from build123d import *

# Parameters (mm, degrees)
SKETCH_1_R      = 2
EXTRUDE_1_DEPTH = 5
FILLET_2_R      = 2


with BuildPart() as part:
    # 草图1 → 凸台-拉伸1 (new body)
    with BuildSketch(Plane.XY):
        with BuildLine():
            Line((-39, -23.5), (39, -23.5))
            Line((39, -23.5), (39, 46.5))
            Line((39, 46.5), (30.3, 46.5))
            Line((30.3, 46.5), (30.3, 29))
            ThreePointArc((30.3, 29), (0, -1.3), (-30.3, 29))
            Line((-30.3, 29), (-30.3, 46.5))
            Line((-30.3, 46.5), (-39, 46.5))
            Line((-39, 46.5), (-39, -23.5))
        make_face()
        with Locations((-34.65, 39)):
            Circle(SKETCH_1_R, mode=Mode.SUBTRACT)
        with Locations((-34.65, 19)):
            Circle(SKETCH_1_R, mode=Mode.SUBTRACT)
        with Locations((34.65, 19)):
            Circle(SKETCH_1_R, mode=Mode.SUBTRACT)
        with Locations((34.65, 39)):
            Circle(SKETCH_1_R, mode=Mode.SUBTRACT)
        with BuildLine():
            Line((-32, -10.5), (-32, -16.5))
            ThreePointArc((-32, -16.5), (-29, -19.5), (-26, -16.5))
            Line((-26, -16.5), (-26, -10.5))
            ThreePointArc((-26, -10.5), (-29, -7.5), (-32, -10.5))
        make_face(mode=Mode.SUBTRACT)
        with BuildLine():
            Line((26, -10.5), (26, -16.5))
            ThreePointArc((26, -16.5), (29, -19.5), (32, -16.5))
            Line((32, -16.5), (32, -10.5))
            ThreePointArc((32, -10.5), (29, -7.5), (26, -10.5))
        make_face(mode=Mode.SUBTRACT)
    extrude(amount=EXTRUDE_1_DEPTH)

    # 圆角2
    fillet_2_edges = [part.edges().sort_by_distance(p)[0] for p in [
        (30.3, 46.5, 2.5),
        (39, 46.5, 2.5),
        (39, -23.5, 2.5),
        (-39, -23.5, 2.5),
        (-39, 46.5, 2.5),
        (-30.3, 46.5, 2.5),
    ]]
    fillet(fillet_2_edges, radius=FILLET_2_R)


solid = part.part
Check sheet for the modelled part. Datum: model origin and axes. Units: mm. A direction names the side the tool comes from. Coordinates: 2 decimals unless noted, no trailing zeros. Write each loop counter-clockwise with the first axis right and the second up, starting at its lowest first coordinate (ties: lowest second). Pieces come first, ordered by that corner, then holes.
Item 1: Cross-section at A-A on y = -12.5. Record the boundary of the cut face in (x, z), then the cut area to 3 significant figures.
Numbers:
outline: (-39, 0) - (-32, 0) - (-32, 5) - (-39, 5) - close; (-26, 0) - (26, 0) - (26, 5) - (-26, 5) - close; (32, 0) - (39, 0) - (39, 5) - (32, 5) - close
area: 330 mm2
Item 2: Access from +Z, -Z, +X, -X, +Y, -Y to the whole of each face (thin tool, end or side, straight path). Record for faces 5 (the face through (38.43, 45.9, 2.54)), 6 (the face through (28.9, -19.5, 2.5)), 7 (the face through (-30.3, 37, 2)).
Numbers:
face 5: +Z, -Z, +X, +Y
face 6: +Z, -Z
face 7: +Z, -Z, +Y
Item 3: Cross-section at B-B on z = 0.8. Record the boundary of the cut face in (x, y).
Numbers:
outline: (-39, -21.5) arc R2 ccw to (-37, -23.5) - (37, -23.5) arc R2 ccw to (39, -21.5) - (39, 44.5) arc R2 ccw to (37, 46.5) - (32.3, 46.5) arc R2 ccw to (30.3, 44.5) - (30.3, 29) arc R30.3 cw to (-30.3, 29) - (-30.3, 44.5) arc R2 ccw to (-32.3, 46.5) - (-37, 46.5) arc R2 ccw to (-39, 44.5) - close; hole circle Ø4 at (-34.65, 19); hole circle Ø4 at (-34.65, 39); hole (-32, -16.5) arc R3 ccw to (-26, -16.5) - (-26, -10.5) arc R3 ccw to (-32, -10.5) - close; hole (26, -16.5) arc R3 ccw to (32, -16.5) - (32, -10.5) arc R3 ccw to (26, -10.5) - close; hole circle Ø4 at (34.65, 19); hole circle Ø4 at (34.65, 39)
Item 4: Scan lines: probe 1 along Y at (x, z) = (-34.65, 3.8); probe 2 along Y at (x, z) = (-33.5, 4.45); probe 3 along Y at (x, z) = (-27, 1). Record each from-to range of solid material in increasing order.
Numbers:
probe 1: y = -23.5 to 17, 21 to 37, 41 to 46.5
probe 2: y = -23.5 to 17.36, 20.64 to 37.36, 40.64 to 46.5
probe 3: y = -23.5 to -18.74, -8.26 to 15.25
Item 5: Mould release check, pull along Y, two halves, no side actions. Record for faces 1 (the face through (-1, -4, 5)), 2 (the face through (-33.6, 20.7, 2.5)), 3 (the face through (-38.4, -22.93, 2.54)), 4 (the face through (-26, -14, 2)): released by +Y, released by -Y, zero draft, split by the parting line, or undercut.
Numbers:
face 1: zero draft
face 2: undercut
face 3: released by -Y
face 4: undercut
Item 6: Cross-section at D-D on x = -29. Record the boundary of the cut face in (y, z), then the cut area to 3 significant figures.
Numbers:
outline: (-23.5, 0) - (-19.5, 0) - (-19.5, 5) - (-23.5, 5) - close; (-7.5, 0) - (20.22, 0) - (20.22, 5) - (-7.5, 5) - close
area: 159 mm2
Item 7: Cross-section at C-C on y = 34. Record the boundary of the cut face in (x, z).
Numbers:
outline: (-39, 0) - (-30.3, 0) - (-30.3, 5) - (-39, 5) - close; (30.3, 0) - (39, 0) - (39, 5) - (30.3, 5) - close
Item 8: Depth check by flat-ended pin: pin 1 Ø2.5 at (x, y) = (34.65, 19) entering from -Z. Enter the tip coordinate at first touch or a pass-through.
Numbers:
pin 1: passes through
